Print and shaded views of the part. All mm, measured from the part's lowest x, y and z. A direction names the side the tool comes from. Round coordinates to 2 decimals unless told otherwise and drop trailing zeros. Order: outer loops, then holes, each group sorted by start corner. A loop starts at its lowest first (then second) coordinate and runs counter-clockwise, first axis right, second up. Notation, with made-up numbers: (-23.75, 46.25) - (17.25, 46.25) arc R32 ccw to (17.25, 78.25) - close; hole circle Ø3 at (24, 7.5). An arc over 180 degrees is marked (long way). Return JSON: item names as keys, results as strings. Group by question number.
Item 1: Drop flat-ended pins along their axis: pin 1 (8 mm diameter, centred on x = 4.5, y = 2.5, fed in from -Z); pin 2 (0.5 mm diameter, centred on x = 39, z = 0.5, fed in from +Y); pin 3 (0.8 mm diameter, centred on y = 1, z = 0.5, fed in from -X). Give the stop position or say it passes through.
Item 2: Tool access for the marked faces 1, 2, 3, 4 and 5: list every direction of +Z, -Z, +X, -X, +Y, -Y with a clear straight run to the whole face (end or side of a thin tool).
Item 3: Saw through at D-D on y = 3.5. State how many separate pieces and enclosed holes the cut face has, and give its area (3 significant figures).
Item 4: Probe probe 1 along Y at (x, z) = (20, 3); probe 2 along Y at (x, z) = (21.5, 3) (1 decimal); probe 3 along Z at (x, y) = (15, 17.5). List the from-to ranges inside material, lowest first.
Item 5: Saw through at C-C on z = 3.25. List the corners of the cut face in (x, y).
Item 6: Two-plate mould, pull along X, no slides. Class the marked faces 6, 7 and 8: released by +X, released by -X, zero draft, split by the parting line, or undercut.
Item 7: Saw through at A-A on x = 20. List the corners of the cut face in (y, z).
Item 8: Saw through at B-B on y = 9. List the corners of the cut face in (x, z).
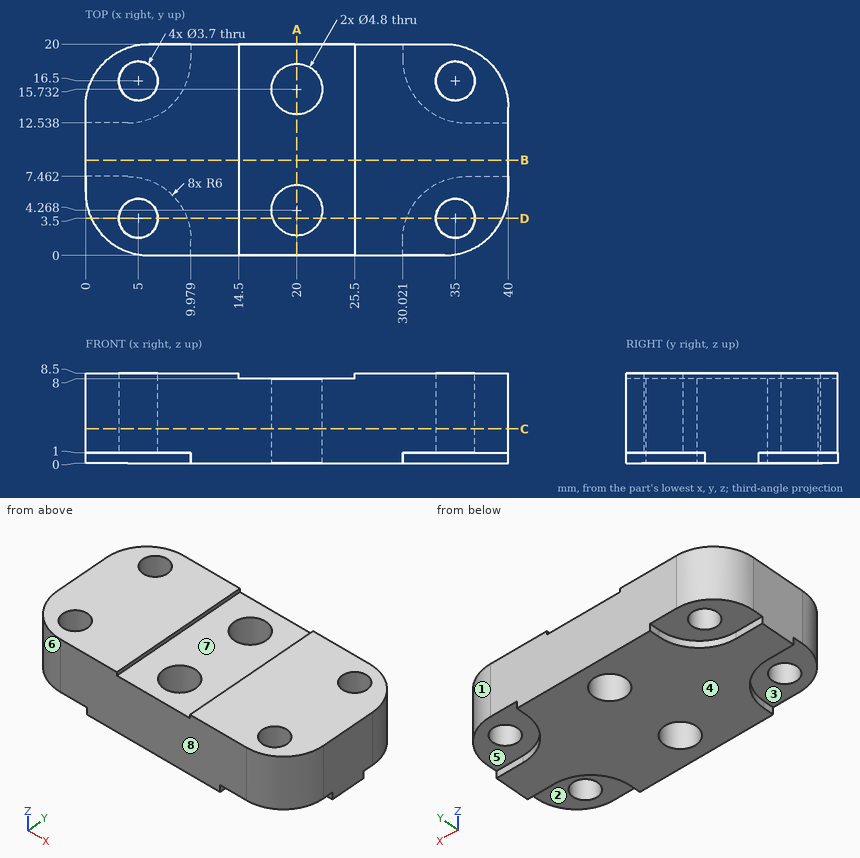
Filled in:
{
 "1": {"pin 1": "stops at z = 1", "pin 2": "stops at y = 12.54", "pin 3": "stops at x = 9.98"},
 "2": {"face 1": "+Z, -Z, +X, +Y", "face 2": "-Z, +X, -Y", "face 3": "-Z, -X, -Y", "face 4": "-Z, +X, -X, +Y, -Y", "face 5": "-Z, +X, +Y"},
 "3": {"separate pieces": "4", "enclosed holes": "0", "area": "215 mm^2"},
 "4": {"probe 1": "y = 0 to 1.87, 6.67 to 13.33, 18.13 to 20", "probe 2": "y = 0 to 2.4, 6.1 to 13.9, 17.6 to 20", "probe 3": "z = 0 to 8"},
 "5": {"outline": "(0, 6) arc R6 ccw to (6, 0) - (34, 0) arc R6 ccw to (40, 6) - (40, 14) arc R6 ccw to (34, 20) - (6, 20) arc R6 ccw to (0, 14) - close; hole circle Ø3.7 at (5, 3.5); hole circle Ø3.7 at (5, 16.5); hole circle Ø4.8 at (20, 4.27); hole circle Ø4.8 at (20, 15.73); hole circle Ø3.7 at (35, 3.5); hole circle Ø3.7 at (35, 16.5)"},
 "6": {"face 6": "released by -X", "face 7": "undercut", "face 8": "zero draft"},
 "7": {"outline": "(0, 0) - (1.87, 0) - (1.87, 8) - (0, 8) - close; (6.67, 0) - (13.33, 0) - (13.33, 8) - (6.67, 8) - close; (18.13, 0) - (20, 0) - (20, 8) - (18.13, 8) - close"},
 "8": {"outline": "(0, 0) - (40, 0) - (40, 8.5) - (25.5, 8.5) - (25.5, 8) - (14.5, 8) - (14.5, 8.5) - (0, 8.5) - close"}
}
